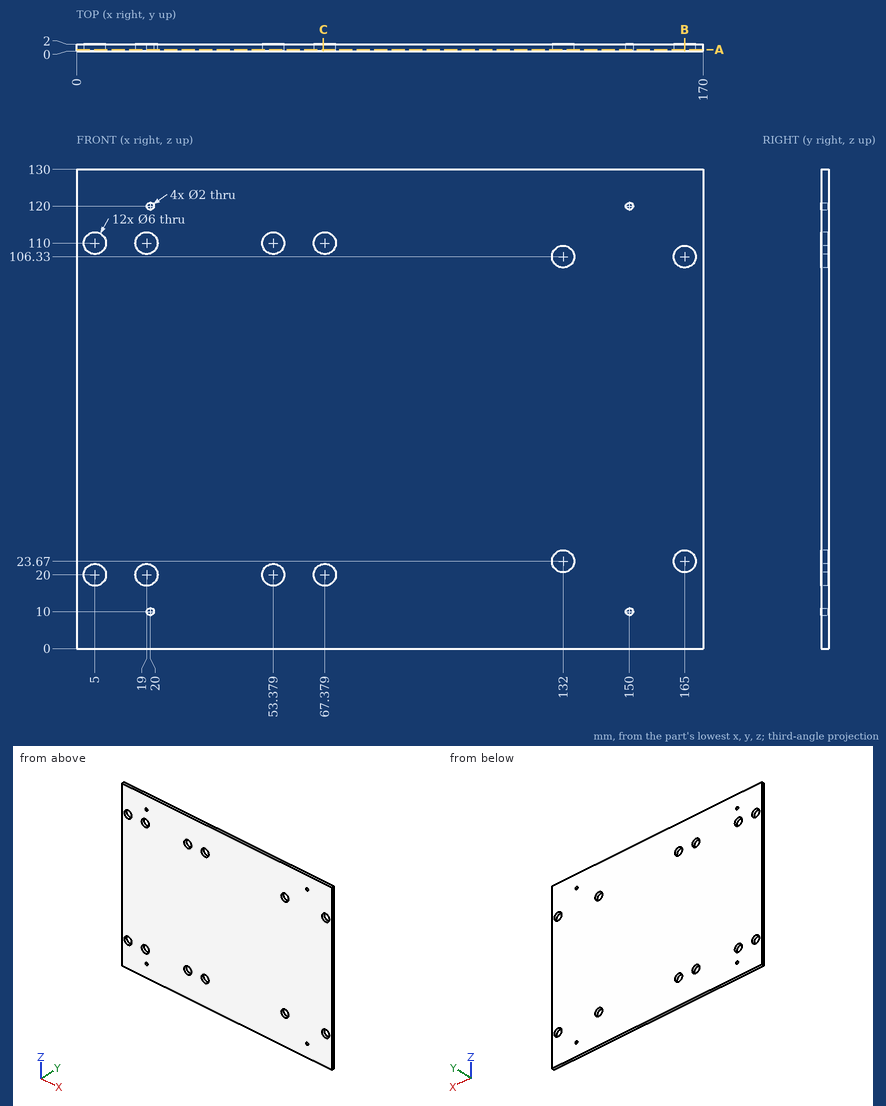
The drawing under review shows one solid part. Ordinate dimensions are in mm from its lowest x, y, z. Give positions to 0.01 mm unless a question says otherwise; leave off trailing zeros. Write each loop counter-clockwise with the first axis right and the second up, starting at its lowest first coordinate (ties: lowest second). Pieces come first, ordered by that corner, then holes. Notation, with made-up numbers: (63, 38) - (107, 38) arc R32 cw to (107, 72) - close; hole circle Ø4 at (39, 5.5). An arc over 180 degrees is marked (long way). Answer in a Markdown table with one row per item. Add a question column.
1. We need section A-A on y = 0.45. State how many separate pieces and enclosed holes the cut face has, then the cut area to 3 significant figures.
2. Wall thickness on line 1 along Z through (x, y) = (67.5, 1.2); line 2 along X through (y, z) = (0.9, 110); line 3 along X through (y, z) = (1.1, 10): over which ranges is each line inside the solid? List them lowest first. Write a range as [from, to].
3. We need section B-B on x = 165. Write out the cut boundary in (y, z).
4. We need section C-C on x = 67. Write out the cut boundary in (y, z), then the cut area to 3 significant figures.
Ans:
| question | item | result |
|---|---|---|
| 1 | separate pieces | 1 |
| 1 | enclosed holes | 16 |
| 1 | area | 21,700 mm^2 |
| 2 | line 1 | z = [0, 17], [23, 107], [113, 130] |
| 2 | line 2 | x = [0, 2], [8, 16], [22, 50.38], [56.38, 64.38], [70.38, 170] |
| 2 | line 3 | x = [0, 19], [21, 149], [151, 170] |
| 3 | outline | (0, 0) - (2, 0) - (2, 20.67) - (0, 20.67) - close; (0, 26.67) - (2, 26.67) - (2, 103.33) - (0, 103.33) - close; (0, 109.33) - (2, 109.33) - (2, 130) - (0, 130) - close |
| 4 | outline | (0, 0) - (2, 0) - (2, 17.02) - (0, 17.02) - close; (0, 22.98) - (2, 22.98) - (2, 107.02) - (0, 107.02) - close; (0, 112.98) - (2, 112.98) - (2, 130) - (0, 130) - close |
| 4 | area | 236 mm^2 |
